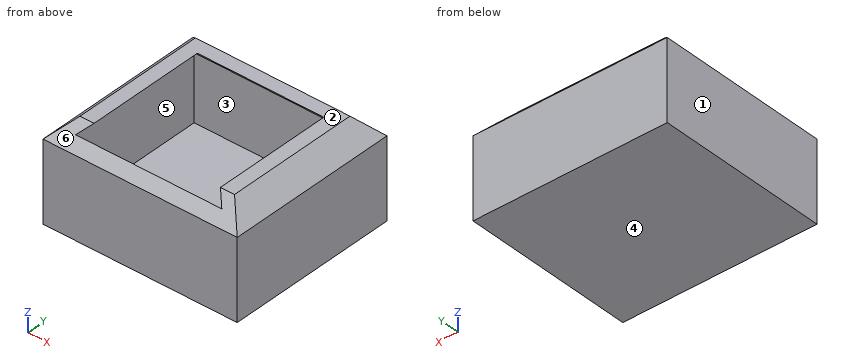
```python
from build123d import *

# Parameters (mm, degrees)
F0_W     = 48.8697811961
F0_H     = 43.6150431633
F1_DEPTH = 25
F2_SIZE  = 5
F3_T     = -2.5


with BuildPart() as f1:
    # F0 (on Top) → F1 (new body)
    with BuildSketch(Plane.XY):
        with Locations((-111.1685223877, 3.0619557947)):
            Rectangle(F0_W, F0_H)
    extrude(amount=F1_DEPTH)

    # F2
    f2_edges = [f1.edges().sort_by_distance(p)[0] for p in [
        (-111.168522, 24.869477, 25),
        (-135.603413, 3.061956, 25),
        (-111.168522, -18.745566, 25),
        (-86.733632, 3.061956, 25),
    ]]
    chamfer(f2_edges, length=F2_SIZE)

    # F3
    f3_openings = [f1.faces().sort_by_distance(p)[0] for p in [
        (-111.168522, -16.340544, 22.405022),
        (-111.168522, 3.061956, 25),
    ]]
    offset(amount=F3_T, openings=f3_openings)


solid = f1.part
```
Geometry: final body of the model. Coordinates: model frame, mm. Face numbers are marked on the shaded views. A direction names the side the tool comes from. Round coordinates to 2 decimals unless told otherwise and drop trailing zeros. Order: outer loops, then holes, each group sorted by start corner. A loop starts at its lowest first (then second) coordinate and runs counter-clockwise, first axis right, second up. Notation, with made-up numbers: (23, 2) -> (76, 2) arc R24 ccw to (76, 36) -> close; hole circle Ø2 at (79, -11). An arc over 180 degrees is marked (long way). Use CSV: the item, a comma, the result in double quotes. Start each with the question number.
1) Material intervals for line 1 along X through (y, z) = (5, 14.75); line 2 along Y through (x, z) = (-116.5, 18); line 3 along Z through (x, y) = (-123.5, -4), sorted ascending. Write a range as from..to.
2) Section B-B (y = 12). Return the cut outline in (x, z), and give its area (3 significant figures).
3) First-contact query: pin 1 Ø1 at (x, y) = (-99, 14) entering from +Z; pin 2 Ø1.5 at (y, z) = (-4.5, 21) entering from +X. Flat tips, straight axial feed; report the tip coordinate or a pass-through.
4) Section A-A (z = 9.5). Return the cut outline in (x, y).
5) Section C-C (x = -109). Return the cut outline in (y, z), and give its area (3 significant figures).
6) Draft query along Z for the marked faces 1, 2, 3 and 4. Return one class per face: +Z half, -Z half, draft (parallel to the pull), parting line (faces both ways), or undercut.
7) Section D-D (y = 21). Return the cut outline in (x, z), and give its area (3 significant figures).
8) Set-up query: the marked faces 5 and 6. Return all of +Z, -Z, +X, -X, +Y, -Y with unobstructed straight access to the full face (end or side cutting, diameter ignored); none if empty.
Returned:
1,line 1,"x = -135.6..-133.1, -89.23..-86.73"
1,line 2,"y = -18.75..-16.25, 22.37..24.87"
1,line 3,"z = 0..2.5"
2,outline,"(-135.6, 0) -> (-86.73, 0) -> (-86.73, 20) -> (-91.73, 25) -> (-95.27, 25) -> (-89.23, 18.96) -> (-89.23, 2.5) -> (-133.1, 2.5) -> (-133.1, 18.96) -> (-127.07, 25) -> (-130.6, 25) -> (-135.6, 20) -> close"
2,area,"246 mm²"
3,pin 1,"stops at z = 2.5"
3,pin 2,"stops at x = -86.98"
4,outline,"(-135.6, -18.75) -> (-86.73, -18.75) -> (-86.73, 24.87) -> (-135.6, 24.87) -> close; hole (-133.1, -16.25) -> (-89.23, -16.25) -> (-89.23, 22.37) -> (-133.1, 22.37) -> close"
5,outline,"(-18.75, 0) -> (24.87, 0) -> (24.87, 20) -> (19.87, 25) -> (16.33, 25) -> (22.37, 18.96) -> (22.37, 2.5) -> (-16.25, 2.5) -> (-16.25, 22.5) -> (-18.75, 20) -> close"
5,area,"218 mm²"
6,face 1,"draft"
6,face 2,"+Z half"
6,face 3,"undercut"
6,face 4,"-Z half"
7,outline,"(-135.6, 0) -> (-86.73, 0) -> (-86.73, 20) -> (-90.6, 23.87) -> (-131.73, 23.87) -> (-135.6, 20) -> close; hole (-133.1, 2.5) -> (-89.23, 2.5) -> (-89.23, 18.96) -> (-90.6, 20.33) -> (-131.73, 20.33) -> (-133.1, 18.96) -> close"
7,area,"371 mm²"
8,face 5,"none"
8,face 6,"+Z, +X, -X, -Y"
